Verification items for the finished model (mm, model axes). Round coordinates to 2 decimals unless told otherwise and drop trailing zeros. Order: outer loops, then holes, each group sorted by start corner. A loop starts at its lowest first (then second) coordinate and runs counter-clockwise, first axis right, second up. Notation, with made-up numbers: M -11,-19.75 L 24,-19.75 A18 cw 24,9.25 Z; hole C 4.5,47 d9. An arc over 180 degrees is marked long. Use CSV: the item, a comma, the result in double quotes. Start each with the question number.
Q1. Gauge pin test, flat ends, axial feed: pin 1 Ø5 at (y, z) = (16.5, 46) entering from -X; pin 2 Ø3 at (y, z) = (22.5, -56) entering from -X; pin 3 Ø2 at (x, z) = (27.5, 33) entering from -Y; pin 4 Ø1 at (y, z) = (6, -62) entering from -X. Record the tip position at first contact, or that the pin passes through.
Q2. Sectioned sample at C-C (y = 21.5). Enter the section's corners in (x, z) (3 decimals), and give its area (3 significant figures).
Q3. Scan lines: line 1 (X direction, y = 13.75, z = 0) (3 decimals); line 2 (Z direction, x = 5.5, y = 18.5). Record each from-to range of solid material in increasing order.
Q4. Sectioned sample at A-A (z = 0). Enter the section's corners in (x, y) (3 decimals), and give its area (3 significant figures).
Q5. Mould release check, pull along Z, two halves, no side actions. Record for faces 1 (the face through (-1, 34.925, -19)), 2 (the face through (46.09, 17.31, -72.28)), 3 (the face through (-3.441, 17.254, 15.497)): +Z half, -Z half, draft (parallel to the pull), parting line (faces both ways), or undercut.
Q6. Sectioned sample at B-B (x = 0). Enter the section's corners in (y, z) (3 decimals).
```python
from build123d import *

# Parameters (mm, degrees)
SKETCH1_R           = 85.725
SKETCH1_R_2         = 15.875
BOSS_EXTRUDE1_DEPTH = 34.925
FILLET1_R           = 6.35
FILLET2_R           = 2.54


with BuildPart() as part:
    # Sketch1 → Boss-Extrude1 (new body)
    with BuildSketch(Plane(origin=(0, 0, 0), x_dir=(1, 0, 0), z_dir=(0, 1, 0))):
        Circle(SKETCH1_R)
        Circle(SKETCH1_R_2, mode=Mode.SUBTRACT)
    extrude(amount=BOSS_EXTRUDE1_DEPTH)

    # Fillet1
    fillet1_edges = [part.edges().sort_by_distance(p)[0] for p in [
        (-85.725, 0, 0),
        (-85.725, 34.925, 0),
    ]]
    fillet(fillet1_edges, radius=FILLET1_R)

    # Fillet2
    fillet2_edges = [part.edges().sort_by_distance(p)[0] for p in [
        (-15.875, 0, 0),
        (-15.875, 34.925, 0),
    ]]
    fillet(fillet2_edges, radius=FILLET2_R)


solid = part.part
```
Verdict:
1,pin 1,"stops at x = -73.87"
1,pin 2,"stops at x = -66.17"
1,pin 3,"stops at y = 0"
1,pin 4,"stops at x = -59.71"
2,outline,"C 0,0 d171.45; hole C 0,0 d31.75"
2,area,"22,300 mm²"
3,line 1,"x = -85.725 to -15.875, 15.875 to 85.725"
3,line 2,"z = -85.55 to -14.89, 14.89 to 85.55"
4,outline,"M -85.725,6.35 A6.35 ccw -79.375,0 L -18.415,0 A2.54 ccw -15.875,2.54 L -15.875,32.385 A2.54 ccw -18.415,34.925 L -79.375,34.925 A6.35 ccw -85.725,28.575 Z; M 15.875,2.54 A2.54 ccw 18.415,0 L 79.375,0 A6.35 ccw 85.725,6.35 L 85.725,28.575 A6.35 ccw 79.375,34.925 L 18.415,34.925 A2.54 ccw 15.875,32.385 Z"
4,area,"4,840 mm²"
5,face 1,"draft"
5,face 2,"parting line"
5,face 3,"undercut"
6,outline,"M 0,-79.375 A6.35 ccw 6.35,-85.725 L 28.575,-85.725 A6.35 ccw 34.925,-79.375 L 34.925,-18.415 A2.54 ccw 32.385,-15.875 L 2.54,-15.875 A2.54 ccw 0,-18.415 Z; M 0,18.415 A2.54 ccw 2.54,15.875 L 32.385,15.875 A2.54 ccw 34.925,18.415 L 34.925,79.375 A6.35 ccw 28.575,85.725 L 6.35,85.725 A6.35 ccw 0,79.375 Z"
